```python
from build123d import *

# Parameters (mm, degrees)
SKETCH1_W           = 132.08
SKETCH1_H           = 144.78
BOSS_EXTRUDE1_DEPTH = 373.38
FILLET1_R           = 17.78
SHELL1_T            = -6.35
SKETCH2_W           = 6.35
SKETCH2_H           = 109.22
BOSS_EXTRUDE2_DEPTH = 55.88
SKETCH3_R           = 6.35
CUT_EXTRUDE1_DEPTH  = 383.54


with BuildPart() as part:
    # Sketch1 → Boss-Extrude1 (new body)
    with BuildSketch(Plane(origin=(0, 0, 0), x_dir=(0, 0, -1), z_dir=(1, 0, 0))):
        with Locations((66.04, 72.39)):
            Rectangle(SKETCH1_W, SKETCH1_H)
    extrude(amount=BOSS_EXTRUDE1_DEPTH)

    # Fillet1
    fillet1_edges = [part.edges().sort_by_distance(p)[0] for p in [
        (373.38, 144.78, -66.04),
        (373.38, 72.39, 0),
        (0, 144.78, -66.04),
        (0, 0, -66.04),
        (0, 72.39, 0),
        (186.69, 144.78, 0),
        (186.69, 0, 0),
        (373.38, 0, -66.04),
    ]]
    fillet(fillet1_edges, radius=FILLET1_R)

    # Shell1
    shell1_openings = [part.faces().sort_by_distance(p)[0] for p in [
        (186.69, 72.39, -132.08),
    ]]
    offset(amount=SHELL1_T, openings=shell1_openings, kind=Kind.INTERSECTION)

    # Sketch2 → Boss-Extrude2 (add)
    with BuildSketch(Plane(origin=(0, 0, -132.08), x_dir=(-1, 0, 0), z_dir=(0, 0, -1))):
        with BuildLine():
            Line((-355.6, 144.78), (-355.6, 138.43))
            ThreePointArc((-355.6, 138.43), (-363.682230509, 135.082230509), (-367.03, 127))
            Line((-367.03, 127), (-373.38, 127))
            ThreePointArc((-373.38, 127), (-368.172358569, 139.572358569), (-355.6, 144.78))
        make_face()
        with Locations((-370.205, 72.39)):
            Rectangle(SKETCH2_W, SKETCH2_H)
        with BuildLine():
            Line((-355.6, 6.35), (-355.6, 0))
            ThreePointArc((-355.6, 0), (-368.172358569, 5.207641431), (-373.38, 17.78))
            Line((-373.38, 17.78), (-367.03, 17.78))
            ThreePointArc((-367.03, 17.78), (-363.682230509, 9.697769491), (-355.6, 6.35))
        make_face()
        with BuildLine():
            Line((-17.78, 138.43), (-17.78, 144.78))
            ThreePointArc((-17.78, 144.78), (-5.207641431, 139.572358569), (0, 127))
            Line((0, 127), (-6.35, 127))
            ThreePointArc((-6.35, 127), (-9.697769491, 135.082230509), (-17.78, 138.43))
        make_face()
        with Locations((-3.175, 72.39)):
            Rectangle(SKETCH2_W, SKETCH2_H)
        with BuildLine():
            Line((-6.35, 17.78), (0, 17.78))
            ThreePointArc((0, 17.78), (-5.207641431, 5.207641431), (-17.78, 0))
            Line((-17.78, 0), (-17.78, 6.35))
            ThreePointArc((-17.78, 6.35), (-9.697769491, 9.697769491), (-6.35, 17.78))
        make_face()
    extrude(amount=BOSS_EXTRUDE2_DEPTH)

    # Sketch3 → Cut-Extrude1 (cut)
    with BuildSketch(Plane(origin=(373.38, 0, 0), x_dir=(0, 0, -1), z_dir=(1, 0, 0))):
        with Locations(Location((170.18, 72.39, 0), (0, 0, 180))):
            Circle(SKETCH3_R)
    extrude(amount=-CUT_EXTRUDE1_DEPTH, mode=Mode.SUBTRACT)


solid = part.part
```
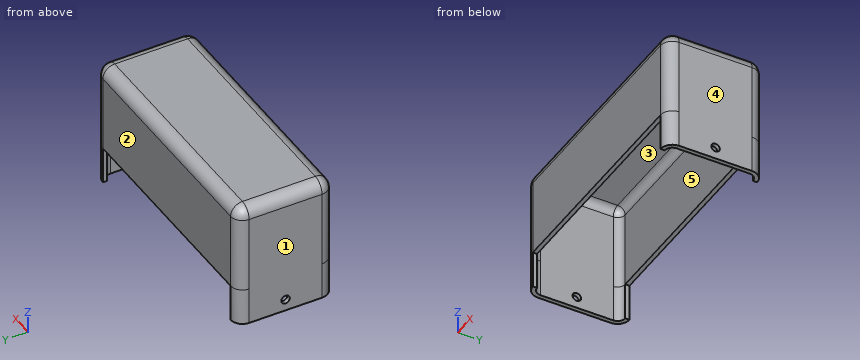
Geometry: final body of the model. Coordinates: model frame, mm. Face numbers are marked on the shaded views. A direction names the side the tool comes from. Coordinates: 2 decimals unless noted, no trailing zeros. Order: outer loops, then holes, each group sorted by start corner. A loop starts at its lowest first (then second) coordinate and runs counter-clockwise, first axis right, second up. Notation, with made-up numbers: (66.25, -3) - (112.25, -3) arc R15 cw to (112.25, 12) - close; hole circle Ø1 at (5.25, 47.25). An arc over 180 degrees is marked (long way). Write each question's results on one line, items separated by ' | '.
(1) First-contact query: pin 1 Ø7 at (y, z) = (4.5, -155) entering from -X; pin 2 Ø1.9 at (y, z) = (142, -161.5) entering from -X; pin 3 Ø7.5 at (y, z) = (72.39, -170.18) entering from -X; pin 4 Ø3 at (x, y) = (205, 3) entering from -Z. Flat tips, straight axial feed; report the tip coordinate or a pass-through.
Values found:
pin 1: stops at x = 2.93 | pin 2: stops at x = 6.88 | pin 3: passes through | pin 4: stops at z = -132.08
(2) Section query B-B, the plane z = -170.18. Return the cut outline in (x, y).
Values found:
outline: (0, 17.78) arc R17.78 ccw to (17.78, 0) - (17.78, 6.35) arc R11.43 cw to (6.35, 17.78) - (6.35, 66.04) - (0, 66.04) - close; (0, 78.74) - (6.35, 78.74) - (6.35, 127) arc R11.43 cw to (17.78, 138.43) - (17.78, 144.78) arc R17.78 ccw to (0, 127) - close; (355.6, 0) arc R17.78 ccw to (373.38, 17.78) - (373.38, 66.04) - (367.03, 66.04) - (367.03, 17.78) arc R11.43 cw to (355.6, 6.35) - close; (355.6, 138.43) arc R11.43 cw to (367.03, 127) - (367.03, 78.74) - (373.38, 78.74) - (373.38, 127) arc R17.78 ccw to (355.6, 144.78) - close
(3) Section query C-C, the plane x = 182. Return the cut outline in (y, z).
Values found:
outline: (0, -132.08) - (6.35, -132.08) - (6.35, -17.78) arc R11.43 cw to (17.78, -6.35) - (127, -6.35) arc R11.43 cw to (138.43, -17.78) - (138.43, -132.08) - (144.78, -132.08) - (144.78, -17.78) arc R17.78 ccw to (127, 0) - (17.78, 0) arc R17.78 ccw to (0, -17.78) - close
(4) Section query A-A, the plane y = 72.39. Return the cut outline in (x, z), plus the area to 3 significant figures.
Values found:
outline: (0, -187.96) - (6.35, -187.96) - (6.35, -176.53) - (0, -176.53) - close; (0, -163.83) - (6.35, -163.83) - (6.35, -17.78) arc R11.43 cw to (17.78, -6.35) - (355.6, -6.35) arc R11.43 cw to (367.03, -17.78) - (367.03, -163.83) - (373.38, -163.83) - (373.38, -17.78) arc R17.78 ccw to (355.6, 0) - (17.78, 0) arc R17.78 ccw to (0, -17.78) - close; (367.03, -187.96) - (373.38, -187.96) - (373.38, -176.53) - (367.03, -176.53) - close | area: 4,440 mm²
(5) Set-up query: the marked faces 4 and 5. Return all of +Z, -Z, +X, -X, +Y, -Y with unobstructed straight access to the full face (end or side cutting, diameter ignored); none if empty.
Values found:
face 4: +Z, -Z, +X, +Y, -Y | face 5: -Z
(6) Line query: line 1 (X direction, y = 39, z = -23); line 2 (Y direction, x = 272, z = -20.5). Output: solid intervals per line, ascending. Write a range as [from, to].
Values found:
line 1: x = [0, 6.35], [367.03, 373.38] | line 2: y = [0, 6.35], [138.43, 144.78]
(7) Section query D-D, the plane z = -58. Return the cut outline in (x, y), plus the area to 3 significant figures.
Values found:
outline: (0, 17.78) arc R17.78 ccw to (17.78, 0) - (355.6, 0) arc R17.78 ccw to (373.38, 17.78) - (373.38, 127) arc R17.78 ccw to (355.6, 144.78) - (17.78, 144.78) arc R17.78 ccw to (0, 127) - close; hole (6.35, 17.78) arc R11.43 ccw to (17.78, 6.35) - (355.6, 6.35) arc R11.43 ccw to (367.03, 17.78) - (367.03, 127) arc R11.43 ccw to (355.6, 138.43) - (17.78, 138.43) arc R11.43 ccw to (6.35, 127) - close | area: 6,260 mm²
(8) Mould query, pull axis X, two halves, no side actions, for the marked faces 1, 2 and 3. Classes: +X half, -X half, draft (parallel to the pull), parting line (faces both ways), or undercut.
Values found:
face 1: -X half | face 2: draft | face 3: undercut
